Part model, mm, in its own coordinate system. A direction names the side the tool comes from. Round coordinates to 2 decimals unless told otherwise and drop trailing zeros. Loops run counter-clockwise (first coordinate to the right, second up) from the corner with the lowest first, then second, coordinate; pieces in that order, holes last.
1) Band-saw the part on D-D, the plane z = 12.7. State how many separate pieces and enclosed holes the cut face has, then the cut area to 3 significant figures.
2) Band-saw the part on B-B, the plane x = -2.5. Write the cut outline in (y, z).
3) Band-saw the part on C-C, the plane z = 34. Write the cut outline in (x, y) (3 decimals).
4) Mould opens along Y. For faces 4 (the cylindrical face through (14.71, 58.94, 13.25)), 5 (the flat face through (15, 69.147, 25)), 6 (the flat face through (-18, -27.373, 25)), 7 (the flat face through (8.086, 21, 26)) say: +Y half, -Y half, draft (parallel to the pull), parting line (faces both ways), or undercut.
5) Band-saw the part on A-A, the plane y = 51.5. Write the cut outline in (x, z), then the cut area to 3 significant figures.
6) Probe line 1 (Y direction, x = -17.75, z = 12.7); line 2 (X direction, y = 63.5, z = 3); line 3 (Y direction, x = -18, z = 12). List the from-to ranges inside material, lowest first.
7) 3-axis set-ups, long thin cutter, end or side, ignore diameter. For faces 1 (the cylindrical face through (-10.06, 30.09, 25.04)), 2 (the flat face through (-14.774, -14, 26)), 3 (the flat face through (-14.774, 57, 26)): which of +Z, -Z, +X, -X, +Y, -Y reach the whole face in a straight line?
8) Drop flat-ended pins along their axis: P1, Ø4.5, axis at y = 56.45, z = 38.1, coming from the -X side; P2, Ø6.5, axis at x = -0.5, z = 15, coming from the +Y side; P3, Ø1, axis at x = 9.5, z = 38.5, coming from the -Y side. Give the stop position or say it passes through.
Autodesk Inventor part; units mm, degrees
ref_plane "YZ Plane" through (0, 0, 0) normal (1, 0, 0) x (0, 1, 0)
ref_plane "XZ Plane" through (0, 0, 0) normal (0, 1, 0) x (-1, 0, 0)
ref_plane "XY Plane" through (0, 0, 0) normal (0, 0, 1) x (1, 0, 0)
sketch "Bracket-CrossArea" plane through (0, 0, 0) normal (0, 0, 1) x (1, 0, 0)
  line L0 (-20.4892, 69.1468) -> (-20.4892, -27.3732)
  line L1 (-20.4892, -27.3732) -> (-14.1392, -27.3732)
  line L2 (-14.1392, -27.3732) -> (-14.1392, -1.9732)
  line L3 (-14.1392, -1.9732) -> (11.2608, -1.9732)
  line L4 (11.2608, -1.9732) -> (11.2608, -27.3732)
  line L5 (11.2608, -27.3732) -> (17.6108, -27.3732)
  line L6 (17.6108, -27.3732) -> (17.6108, 69.1468)
  line L7 (17.6108, 69.1468) -> (11.2608, 69.1468)
  line L8 (11.2608, 69.1468) -> (11.2608, 43.7468)
  line L9 (11.2608, 43.7468) -> (-14.1392, 43.7468)
  line L10 (-14.1392, 43.7468) -> (-14.1392, 69.1468)
  line L11 (-20.4892, 69.1468) -> (-14.1392, 69.1468)
  point P0 (0, 0)
  dimension "d3" = 6.35
  dimension "d4" = 96.52
  dimension "d5" = 25.4
  dimension "d6" = 25.4
  dimension "d7" = 6.35
  dimension "d10" = 25.4
extrude "HBracket_3DShape" add sketch "Bracket-CrossArea" along normal blind 50.8
sketch "Sketch2" plane through (0, 0, 50.8) normal (0, 0, 1) x (1, 0, 0)
  line L0 (-10.9642, 31.0468) -> (8.0858, 31.0468)
  line L1 (8.0858, 31.0468) -> (8.0858, 10.7268)
  line L2 (8.0858, 10.7268) -> (-10.9642, 10.7268)
  line L3 (-10.9642, 10.7268) -> (-10.9642, 31.0468)
  line L4 (11.2608, 43.7468) -> (-14.1392, 43.7468)
  line L5 (-14.1392, -1.9732) -> (11.2608, -1.9732)
  line L6 (-14.1392, 43.7468) -> (-14.1392, 69.1468)
  line L7 (11.2608, 69.1468) -> (11.2608, 43.7468)
  line L8 (17.6108, -27.3732) -> (17.6108, 69.1468)
  line L9 (-20.4892, 69.1468) -> (-20.4892, -27.3732)
  point P0 (0, 0)
  dimension "d11" = 12.7
  dimension "d12" = 12.7
  dimension "d29" = 9.525
  dimension "d30" = 9.525
extrude "MiddleHole" cut sketch "Sketch2" against normal through all
fillet "RoundedInside" radius 3.175 4 edges at (-10.9642, 10.7268, 25.4) (-10.9642, 31.0468, 25.4) (8.0858, 31.0468, 25.4) (8.0858, 10.7268, 25.4)
sketch "Sketch4" plane through (17.6108, -27.3732, 0) normal (1, 0, 0) x (0, 0, -1)
  line L0 (0, 71.12) -> (-50.8, 71.12)
  line L1 (0, 71.12) -> (-50.8, 71.12)
  line L2 (0, 0) -> (-50.8, 0)
  line L3 (0, 25.4) -> (-50.8, 25.4)
  line L4 (0, 0) -> (0, 96.52)
  line L5 (0, 96.52) -> (-50.8, 96.52)
  line L6 (-50.8, 0) -> (-50.8, 96.52)
  line L7 (0, 0) -> (-50.8, 0)
  point P0 (0, 27.3732)
  point P1 (-38.1, 83.82)
  point P2 (-12.7, 83.82)
  point P3 (-38.1, 12.7)
  point P4 (-12.7, 12.7)
  dimension "d48" = 12.7
  dimension "d49" = 12.7
  dimension "d52" = 25.4
  dimension "d55" = 71.12
hole "Screw Holes" at (17.6108, 56.4468, 38.1) at (17.6108, 56.4468, 12.7) at (17.6108, -14.6732, 38.1) at (17.6108, -14.6732, 12.7) direction (-1, 0, 0) diameter 5.1054 end through all
sketch "GapSpacing" plane through (0, 0, 50.8) normal (0, 0, 1) x (1, 0, 0)
  line L0 (-20.4892, -27.3732) -> (-14.1392, -27.3732)
  line L1 (-14.1392, -27.3732) -> (-14.1392, -1.9732)
  line L2 (-14.1392, -1.9732) -> (11.2608, -1.9732)
  line L3 (11.2608, -1.9732) -> (11.2608, -27.3732)
  line L4 (11.2608, -27.3732) -> (17.6108, -27.3732)
  line L5 (17.6108, -27.3732) -> (17.6108, 69.1468)
  line L6 (17.6108, 69.1468) -> (11.2608, 69.1468)
  line L7 (11.2608, 69.1468) -> (11.2608, 43.7468)
  line L8 (11.2608, 43.7468) -> (-14.1392, 43.7468)
  line L9 (-14.1392, 43.7468) -> (-14.1392, 69.1468)
  line L10 (-14.1392, 69.1468) -> (-20.4892, 69.1468)
  line L11 (-20.4892, 69.1468) -> (-20.4892, -27.3732)
  line L12 (-14.7742, 43.7468) -> (11.8958, 43.7468)
  line L13 (11.8958, 43.7468) -> (11.8958, 73.025)
  line L14 (11.8958, 73.025) -> (-14.7742, 73.025)
  line L15 (-14.7742, 73.025) -> (-14.7742, 43.7468)
  line L16 (-14.7742, -30.1625) -> (11.8958, -30.1625)
  line L17 (11.8958, -30.1625) -> (11.8958, -1.9732)
  line L18 (11.8958, -1.9732) -> (-14.7742, -1.9732)
  line L19 (-14.7742, -1.9732) -> (-14.7742, -30.1625)
  point P0 (-14.7742, -27.3732)
  point P1 (11.8958, -27.3732)
  point P2 (11.8958, 69.1468)
  point P3 (-14.7742, 69.1468)
  point P4 (-14.1392, 43.7468)
  point P5 (-14.1392, 43.7468)
  dimension "d58" = 0.635
  dimension "d59" = 0.635
  dimension "d62" = 0.635
  dimension "d63" = 0.635
extrude "GapSpace" cut sketch "GapSpacing" against normal through all contours L19 L18 L1 L0 | L0 L1 L2 L3 L4 L17 L16 L19 | L15 L14 L13 L6 L7 L8 L9 L10 | L10 L9 L12 L15 | L18 L17 L4 L3 | L7 L6 L13 L12
equation "\"d6\" = d5"
equation "\"d7\" = d3"
equation "\"d12\" = d11"
equation "\"d30\" = d29"
equation "\"d59\" = d58"
equation "\"d62\" = d58"
equation "\"d63\" = d58"
properties part number "Arm_H-Bracket"
Reported:
1. separate pieces: 5
1. enclosed holes: 1
1. area: 1,830 mm2
2. outline: (-1.97, 0) - (10.73, 0) - (10.73, 50.8) - (-1.97, 50.8) - close; (31.05, 0) - (43.75, 0) - (43.75, 50.8) - (31.05, 50.8) - close
3. outline: (-20.489, -27.373) - (-14.774, -27.373) - (-14.774, -1.973) - (11.896, -1.973) - (11.896, -27.373) - (17.611, -27.373) - (17.611, 69.147) - (11.896, 69.147) - (11.896, 43.747) - (-14.774, 43.747) - (-14.774, 69.147) - (-20.489, 69.147) - close; hole (-10.964, 13.902) arc R3.175 ccw to (-7.789, 10.727) - (4.911, 10.727) arc R3.175 ccw to (8.086, 13.902) - (8.086, 27.872) arc R3.175 ccw to (4.911, 31.047) - (-7.789, 31.047) arc R3.175 ccw to (-10.964, 27.872) - close
4. face 4: undercut
4. face 5: +Y half
4. face 6: -Y half
4. face 7: undercut
5. outline: (-20.49, 0) - (-14.77, 0) - (-14.77, 50.8) - (-20.49, 50.8) - close; (11.9, 0) - (17.61, 0) - (17.61, 50.8) - (11.9, 50.8) - close
5. area: 581 mm2
6. line 1: y = -27.37 to -17.23, -12.12 to 53.89, 59 to 69.15
6. line 2: x = -20.49 to -14.77, 11.9 to 17.61
6. line 3: y = -27.37 to -17.13, -12.22 to 53.99, 58.9 to 69.15
7. face 1: +Z, -Z
7. face 2: +Z, -Z, -Y
7. face 3: +Z, -Z, +Y
8. P1: passes through
8. P2: stops at y = 43.75
8. P3: stops at y = -1.97
